Build history of the part. All positions in model axes, mm. Round coordinates to 2 decimals unless told otherwise and drop trailing zeros. Write each loop counter-clockwise with the first axis right and the second up, starting at its lowest first coordinate (ties: lowest second). Pieces come first, ordered by that corner, then holes.
Item 1: Band-saw the part on D-D, the plane x = -38.5. Write the cut outline in (y, z).
Item 2: Band-saw the part on A-A, the plane y = -7. Write the cut outline in (x, z).
Item 3: Band-saw the part on C-C, the plane z = 2.5. Count the separate pieces of the cut face and the enclosed holes in it, then the cut area to 3 significant figures.
Item 4: Wall check: probe 1 along Y at (x, z) = (-45, 2); probe 2 along X at (y, z) = (1.5, 1.9); probe 3 along Y at (x, z) = (0, 1.7). Give the ranges that are in metal, low to high.
Item 5: Band-saw the part on B-B, the plane x = 23. Write the cut outline in (y, z), then the cut area to 3 significant figures.
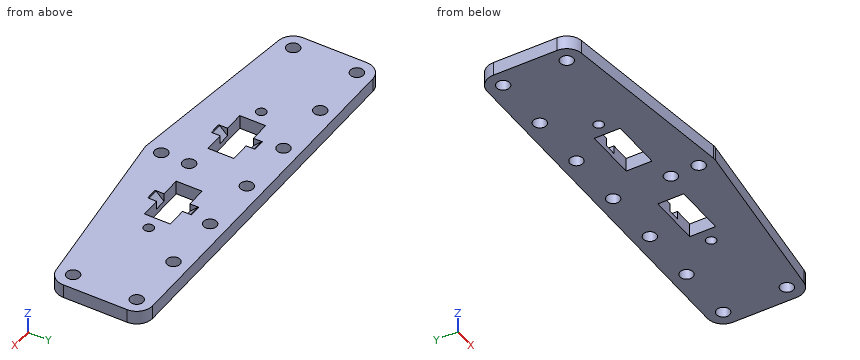
```python
from build123d import *

# Parameters (mm, degrees)
SZKIC1_R                    = 1.65
DODANIE_WYCI_GNI_CIE1_DEPTH = 3.5
SZKIC2_W                    = 13
SZKIC2_H                    = 6.5
WYTNIJ_WYCI_GNI_CIE1_DEPTH  = 4
SZKIC3_R                    = 1.25
WYTNIJ_WYCI_GNI_CIE2_DEPTH  = 4
SZKIC4_R                    = 1.65
WYTNIJ_WYCI_GNI_CIE3_DEPTH  = 4
SZKIC5_W                    = 3
SZKIC5_H                    = 11
WYTNIJ_WYCI_GNI_CIE4_DEPTH  = 0.1
SFAZOWANIE1_SIZE            = 2
SFAZOWANIE2_SIZE            = 2


with BuildPart() as part:
    # Szkic1 → Dodanie-wyciągnięcie1 (new body)
    with BuildSketch(Plane.XY):
        with BuildLine():
            ThreePointArc((-0.48527772, -10.970454072), (0, -11), (0.48527772, -10.970454072))
            Line((0.48527772, -10.970454072), (45.48527772, -5.470454072))
            ThreePointArc((45.48527772, -5.470454072), (47.995088553, -4.151309971), (49, -1.5))
            Line((49, -1.5), (49, 14.5))
            ThreePointArc((49, 14.5), (47.828427125, 17.328427125), (45, 18.5))
            Line((45, 18.5), (-45, 18.5))
            ThreePointArc((-45, 18.5), (-47.828427125, 17.328427125), (-49, 14.5))
            Line((-49, 14.5), (-49, -1.5))
            ThreePointArc((-49, -1.5), (-47.995088553, -4.151309971), (-45.48527772, -5.470454072))
            Line((-45.48527772, -5.470454072), (-0.48527772, -10.970454072))
        make_face()
        with Locations((0, -7)):
            Circle(SZKIC1_R, mode=Mode.SUBTRACT)
        with Locations((-45, -1.5)):
            Circle(SZKIC1_R, mode=Mode.SUBTRACT)
        Circle(SZKIC1_R, mode=Mode.SUBTRACT)
        with Locations((45, -1.5)):
            Circle(SZKIC1_R, mode=Mode.SUBTRACT)
        with Locations((-45, 14.5)):
            Circle(SZKIC1_R, mode=Mode.SUBTRACT)
        with Locations((45, 14.5)):
            Circle(SZKIC1_R, mode=Mode.SUBTRACT)
    extrude(amount=DODANIE_WYCI_GNI_CIE1_DEPTH)

    # Szkic2 → Wytnij-wyciągnięcie1 (cut)
    with BuildSketch(Plane.XY.offset(3.5)):
        with Locations((13, 4)):
            Rectangle(SZKIC2_W, SZKIC2_H)
    wytnij_wyci_gni_cie1 = extrude(amount=-WYTNIJ_WYCI_GNI_CIE1_DEPTH, mode=Mode.SUBTRACT)

    # Szkic3 → Wytnij-wyciągnięcie2 (cut)
    with BuildSketch(Plane.XY.offset(3.5)):
        with Locations((23, 4)):
            Circle(SZKIC3_R)
    wytnij_wyci_gni_cie2 = extrude(amount=-WYTNIJ_WYCI_GNI_CIE2_DEPTH, mode=Mode.SUBTRACT)

    # Lustro1: Wytnij-wyciągnięcie1, Wytnij-wyciągnięcie2 across plane
    add(wytnij_wyci_gni_cie1.mirror(Plane(origin=(0, 0, 0), x_dir=(0, 0, 1), z_dir=(1, 0, 0))), mode=Mode.SUBTRACT)
    add(wytnij_wyci_gni_cie2.mirror(Plane(origin=(0, 0, 0), x_dir=(0, 0, 1), z_dir=(1, 0, 0))), mode=Mode.SUBTRACT)

    # Szkic4 → Wytnij-wyciągnięcie3 (cut)
    with BuildSketch(Plane.XY.offset(3.5)):
        with Locations((0, 14.5)):
            Circle(SZKIC4_R)
        with Locations((15, 14.5)):
            Circle(SZKIC4_R)
        with Locations((30, 14.5)):
            Circle(SZKIC4_R)
    wytnij_wyci_gni_cie3 = extrude(amount=-WYTNIJ_WYCI_GNI_CIE3_DEPTH, mode=Mode.SUBTRACT)

    # Lustro2: Wytnij-wyciągnięcie3 across plane
    add(wytnij_wyci_gni_cie3.mirror(Plane(origin=(0, 0, 0), x_dir=(0, 0, 1), z_dir=(1, 0, 0))), mode=Mode.SUBTRACT)

    # Szkic5 → Wytnij-wyciągnięcie4 (cut)
    with BuildSketch(Plane.XY.offset(3.5)):
        with Locations((13, 4)):
            Rectangle(SZKIC5_W, SZKIC5_H)
    wytnij_wyci_gni_cie4 = extrude(amount=-WYTNIJ_WYCI_GNI_CIE4_DEPTH, mode=Mode.SUBTRACT)

    # Sfazowanie1
    sfazowanie1_edges = [part.edges().sort_by_distance(p)[0] for p in [
        (13, 7.25, 3.4),
        (13, 0.75, 3.4),
    ]]
    chamfer(sfazowanie1_edges, length=SFAZOWANIE1_SIZE)

    # Lustro6: Wytnij-wyciągnięcie4 across plane
    add(wytnij_wyci_gni_cie4.mirror(Plane(origin=(0, 0, 0), x_dir=(0, 0, 1), z_dir=(1, 0, 0))), mode=Mode.SUBTRACT)

    # Sfazowanie2
    sfazowanie2_edges = [part.edges().sort_by_distance(p)[0] for p in [
        (-13, 0.75, 3.4),
        (-13, 7.25, 3.4),
    ]]
    chamfer(sfazowanie2_edges, length=SFAZOWANIE2_SIZE)


solid = part.part
```
Results:
1. outline: (-6.32, 0) - (18.5, 0) - (18.5, 3.5) - (-6.32, 3.5) - close
2. outline: (-32.97, 0) - (-1.65, 0) - (-1.65, 3.5) - (-32.97, 3.5) - close; (1.65, 0) - (32.97, 0) - (32.97, 3.5) - (1.65, 3.5) - close
3. separate pieces: 1
3. enclosed holes: 15
3. area: 2,300 mm2
4. probe 1: y = -5.53 to -3.15, 0.15 to 12.85, 16.15 to 18.5
4. probe 2: x = -49 to -19.5, -6.5 to -0.69, 0.69 to 6.5, 19.5 to 49
4. probe 3: y = -11 to -8.65, -5.35 to -1.65, 1.65 to 12.85, 16.15 to 18.5
5. outline: (-8.22, 0) - (2.75, 0) - (2.75, 3.5) - (-8.22, 3.5) - close; (5.25, 0) - (18.5, 0) - (18.5, 3.5) - (5.25, 3.5) - close
5. area: 84.8 mm2
